Could you check a few things on this model? Use its own coordinates, in mm. A direction names the side the tool comes from. Give positions to 0.01 mm unless a question says otherwise; leave off trailing zeros. Order: outer loops, then holes, each group sorted by start corner. A loop starts at its lowest first (then second) coordinate and runs counter-clockwise, first axis right, second up.
from build123d import *

# Parameters (mm, degrees)
ESQUISSE1_W                                    = 408.5
ESQUISSE1_H                                    = 181
BOSS_EXTRU_1_DEPTH                             = 8
CHAMBRAGE_POUR_VIS_T_TE_RONDE_BOMB_2_COUNT     = 2
CHAMBRAGE_POUR_VIS_T_TE_RONDE_BOMB_2_PITCH     = 56
CHAMBRAGE_POUR_VIS_T_TE_RONDE_BOMB_3_COUNT     = 2
CHAMBRAGE_POUR_VIS_T_TE_RONDE_BOMB_3_PITCH     = 140
R_P_TITION_LIN_AIRE1_COUNT                     = 11
R_P_TITION_LIN_AIRE1_PITCH                     = 33
ESQUISSE4_W                                    = 22.5
ESQUISSE4_H                                    = 4.5
ENL_V_MAT_EXTRU_1_DEPTH                        = 181
ESQUISSE5_W                                    = 22.5
ESQUISSE5_H                                    = 18.725
BOSS_EXTRU_2_DEPTH                             = 3.5
ESQUISSE7_W                                    = 274.5
ESQUISSE7_H                                    = 22.375
BOSS_EXTRU_3_DEPTH                             = 5
FRAISAGE_POUR_VIS_T_TE_FRAIS_E_M31_D           = 3.4
FRAISAGE_POUR_VIS_T_TE_FRAIS_E_M31_CSINK_D     = 6.3
FRAISAGE_POUR_VIS_T_TE_FRAIS_E_M31_CSINK_ANGLE = 90


with BuildPart() as part:
    # Esquisse1 → Boss.-Extru.1 (new body)
    with BuildSketch(Plane.XY):
        Rectangle(ESQUISSE1_W, ESQUISSE1_H)
    extrude(amount=BOSS_EXTRU_1_DEPTH)

    # Esquisse3 → Chambrage pour vis à tête ronde bombée M31 (revolve, cut)
    with BuildSketch(Plane(origin=(-156.75, 63, 8), x_dir=(0, -1, 0), z_dir=(1, 0, 0))):
        Polygon((0, 0), (0, 8), (1.6, 8), (1.6, 2.4), (3.5, 2.4), (3.5, 0.025), (3.525, 0), align=None)
    chambrage_pour_vis_t_te_ronde_bomb_e_m = revolve(axis=Axis((-156.75, 63, 14.35), (0, 0, -1)), mode=Mode.SUBTRACT)

    # Chambrage pour vis _ t_te ronde bomb 2: Chambrage pour vis à tête ronde bombée M31 ×2
    with Locations(*[(0, -i * CHAMBRAGE_POUR_VIS_T_TE_RONDE_BOMB_2_PITCH, 0) for i in range(1, CHAMBRAGE_POUR_VIS_T_TE_RONDE_BOMB_2_COUNT)]):
        add(chambrage_pour_vis_t_te_ronde_bomb_e_m, mode=Mode.SUBTRACT)

    # Chambrage pour vis _ t_te ronde bomb 3: Chambrage pour vis à tête ronde bombée M31 ×2
    with Locations(*[(0, -i * CHAMBRAGE_POUR_VIS_T_TE_RONDE_BOMB_3_PITCH, 0) for i in range(1, CHAMBRAGE_POUR_VIS_T_TE_RONDE_BOMB_3_COUNT)]):
        add(chambrage_pour_vis_t_te_ronde_bomb_e_m, mode=Mode.SUBTRACT)

    # Répétition linéaire1: Chambrage pour vis à tête ronde bombée M31 ×11
    with Locations(*[(i * R_P_TITION_LIN_AIRE1_PITCH, 0, 0) for i in range(1, R_P_TITION_LIN_AIRE1_COUNT)]):
        add(chambrage_pour_vis_t_te_ronde_bomb_e_m, mode=Mode.SUBTRACT)

    # Répétition linéaire1 copy 1 sketch → Répétition linéaire1 copy 1 (revolve, cut)
    with BuildSketch(Plane(origin=(-123.75, 7, 8), x_dir=(0, -1, 0), z_dir=(1, 0, 0))):
        Polygon((0, 0), (0, 8), (1.6, 8), (1.6, 2.4), (3.5, 2.4), (3.5, 0.025), (3.525, 0), align=None)
    revolve(axis=Axis((-123.75, 7, 14.35), (0, 0, -1)), mode=Mode.SUBTRACT)

    # Répétition linéaire1 copy 2 sketch → Répétition linéaire1 copy 2 (revolve, cut)
    with BuildSketch(Plane(origin=(-90.75, 7, 8), x_dir=(0, -1, 0), z_dir=(1, 0, 0))):
        Polygon((0, 0), (0, 8), (1.6, 8), (1.6, 2.4), (3.5, 2.4), (3.5, 0.025), (3.525, 0), align=None)
    revolve(axis=Axis((-90.75, 7, 14.35), (0, 0, -1)), mode=Mode.SUBTRACT)

    # Répétition linéaire1 copy 3 sketch → Répétition linéaire1 copy 3 (revolve, cut)
    with BuildSketch(Plane(origin=(-57.75, 7, 8), x_dir=(0, -1, 0), z_dir=(1, 0, 0))):
        Polygon((0, 0), (0, 8), (1.6, 8), (1.6, 2.4), (3.5, 2.4), (3.5, 0.025), (3.525, 0), align=None)
    revolve(axis=Axis((-57.75, 7, 14.35), (0, 0, -1)), mode=Mode.SUBTRACT)

    # Répétition linéaire1 copy 4 sketch → Répétition linéaire1 copy 4 (revolve, cut)
    with BuildSketch(Plane(origin=(-24.75, 7, 8), x_dir=(0, -1, 0), z_dir=(1, 0, 0))):
        Polygon((0, 0), (0, 8), (1.6, 8), (1.6, 2.4), (3.5, 2.4), (3.5, 0.025), (3.525, 0), align=None)
    revolve(axis=Axis((-24.75, 7, 14.35), (0, 0, -1)), mode=Mode.SUBTRACT)

    # Répétition linéaire1 copy 5 sketch → Répétition linéaire1 copy 5 (revolve, cut)
    with BuildSketch(Plane(origin=(8.25, 7, 8), x_dir=(0, -1, 0), z_dir=(1, 0, 0))):
        Polygon((0, 0), (0, 8), (1.6, 8), (1.6, 2.4), (3.5, 2.4), (3.5, 0.025), (3.525, 0), align=None)
    revolve(axis=Axis((8.25, 7, 14.35), (0, 0, -1)), mode=Mode.SUBTRACT)

    # Répétition linéaire1 copy 6 sketch → Répétition linéaire1 copy 6 (revolve, cut)
    with BuildSketch(Plane(origin=(41.25, 7, 8), x_dir=(0, -1, 0), z_dir=(1, 0, 0))):
        Polygon((0, 0), (0, 8), (1.6, 8), (1.6, 2.4), (3.5, 2.4), (3.5, 0.025), (3.525, 0), align=None)
    revolve(axis=Axis((41.25, 7, 14.35), (0, 0, -1)), mode=Mode.SUBTRACT)

    # Répétition linéaire1 copy 7 sketch → Répétition linéaire1 copy 7 (revolve, cut)
    with BuildSketch(Plane(origin=(74.25, 7, 8), x_dir=(0, -1, 0), z_dir=(1, 0, 0))):
        Polygon((0, 0), (0, 8), (1.6, 8), (1.6, 2.4), (3.5, 2.4), (3.5, 0.025), (3.525, 0), align=None)
    revolve(axis=Axis((74.25, 7, 14.35), (0, 0, -1)), mode=Mode.SUBTRACT)

    # Répétition linéaire1 copy 8 sketch → Répétition linéaire1 copy 8 (revolve, cut)
    with BuildSketch(Plane(origin=(107.25, 7, 8), x_dir=(0, -1, 0), z_dir=(1, 0, 0))):
        Polygon((0, 0), (0, 8), (1.6, 8), (1.6, 2.4), (3.5, 2.4), (3.5, 0.025), (3.525, 0), align=None)
    revolve(axis=Axis((107.25, 7, 14.35), (0, 0, -1)), mode=Mode.SUBTRACT)

    # Répétition linéaire1 copy 9 sketch → Répétition linéaire1 copy 9 (revolve, cut)
    with BuildSketch(Plane(origin=(140.25, 7, 8), x_dir=(0, -1, 0), z_dir=(1, 0, 0))):
        Polygon((0, 0), (0, 8), (1.6, 8), (1.6, 2.4), (3.5, 2.4), (3.5, 0.025), (3.525, 0), align=None)
    revolve(axis=Axis((140.25, 7, 14.35), (0, 0, -1)), mode=Mode.SUBTRACT)

    # Répétition linéaire1 copy 10 sketch → Répétition linéaire1 copy 10 (revolve, cut)
    with BuildSketch(Plane(origin=(173.25, 7, 8), x_dir=(0, -1, 0), z_dir=(1, 0, 0))):
        Polygon((0, 0), (0, 8), (1.6, 8), (1.6, 2.4), (3.5, 2.4), (3.5, 0.025), (3.525, 0), align=None)
    revolve(axis=Axis((173.25, 7, 14.35), (0, 0, -1)), mode=Mode.SUBTRACT)

    # Répétition linéaire1 copy 11 sketch → Répétition linéaire1 copy 11 (revolve, cut)
    with BuildSketch(Plane(origin=(-123.75, -77, 8), x_dir=(0, -1, 0), z_dir=(1, 0, 0))):
        Polygon((0, 0), (0, 8), (1.6, 8), (1.6, 2.4), (3.5, 2.4), (3.5, 0.025), (3.525, 0), align=None)
    revolve(axis=Axis((-123.75, -77, 14.35), (0, 0, -1)), mode=Mode.SUBTRACT)

    # Répétition linéaire1 copy 12 sketch → Répétition linéaire1 copy 12 (revolve, cut)
    with BuildSketch(Plane(origin=(-90.75, -77, 8), x_dir=(0, -1, 0), z_dir=(1, 0, 0))):
        Polygon((0, 0), (0, 8), (1.6, 8), (1.6, 2.4), (3.5, 2.4), (3.5, 0.025), (3.525, 0), align=None)
    revolve(axis=Axis((-90.75, -77, 14.35), (0, 0, -1)), mode=Mode.SUBTRACT)

    # Répétition linéaire1 copy 13 sketch → Répétition linéaire1 copy 13 (revolve, cut)
    with BuildSketch(Plane(origin=(-57.75, -77, 8), x_dir=(0, -1, 0), z_dir=(1, 0, 0))):
        Polygon((0, 0), (0, 8), (1.6, 8), (1.6, 2.4), (3.5, 2.4), (3.5, 0.025), (3.525, 0), align=None)
    revolve(axis=Axis((-57.75, -77, 14.35), (0, 0, -1)), mode=Mode.SUBTRACT)

    # Répétition linéaire1 copy 14 sketch → Répétition linéaire1 copy 14 (revolve, cut)
    with BuildSketch(Plane(origin=(-24.75, -77, 8), x_dir=(0, -1, 0), z_dir=(1, 0, 0))):
        Polygon((0, 0), (0, 8), (1.6, 8), (1.6, 2.4), (3.5, 2.4), (3.5, 0.025), (3.525, 0), align=None)
    revolve(axis=Axis((-24.75, -77, 14.35), (0, 0, -1)), mode=Mode.SUBTRACT)

    # Répétition linéaire1 copy 15 sketch → Répétition linéaire1 copy 15 (revolve, cut)
    with BuildSketch(Plane(origin=(8.25, -77, 8), x_dir=(0, -1, 0), z_dir=(1, 0, 0))):
        Polygon((0, 0), (0, 8), (1.6, 8), (1.6, 2.4), (3.5, 2.4), (3.5, 0.025), (3.525, 0), align=None)
    revolve(axis=Axis((8.25, -77, 14.35), (0, 0, -1)), mode=Mode.SUBTRACT)

    # Répétition linéaire1 copy 16 sketch → Répétition linéaire1 copy 16 (revolve, cut)
    with BuildSketch(Plane(origin=(41.25, -77, 8), x_dir=(0, -1, 0), z_dir=(1, 0, 0))):
        Polygon((0, 0), (0, 8), (1.6, 8), (1.6, 2.4), (3.5, 2.4), (3.5, 0.025), (3.525, 0), align=None)
    revolve(axis=Axis((41.25, -77, 14.35), (0, 0, -1)), mode=Mode.SUBTRACT)

    # Répétition linéaire1 copy 17 sketch → Répétition linéaire1 copy 17 (revolve, cut)
    with BuildSketch(Plane(origin=(74.25, -77, 8), x_dir=(0, -1, 0), z_dir=(1, 0, 0))):
        Polygon((0, 0), (0, 8), (1.6, 8), (1.6, 2.4), (3.5, 2.4), (3.5, 0.025), (3.525, 0), align=None)
    revolve(axis=Axis((74.25, -77, 14.35), (0, 0, -1)), mode=Mode.SUBTRACT)

    # Répétition linéaire1 copy 18 sketch → Répétition linéaire1 copy 18 (revolve, cut)
    with BuildSketch(Plane(origin=(107.25, -77, 8), x_dir=(0, -1, 0), z_dir=(1, 0, 0))):
        Polygon((0, 0), (0, 8), (1.6, 8), (1.6, 2.4), (3.5, 2.4), (3.5, 0.025), (3.525, 0), align=None)
    revolve(axis=Axis((107.25, -77, 14.35), (0, 0, -1)), mode=Mode.SUBTRACT)

    # Répétition linéaire1 copy 19 sketch → Répétition linéaire1 copy 19 (revolve, cut)
    with BuildSketch(Plane(origin=(140.25, -77, 8), x_dir=(0, -1, 0), z_dir=(1, 0, 0))):
        Polygon((0, 0), (0, 8), (1.6, 8), (1.6, 2.4), (3.5, 2.4), (3.5, 0.025), (3.525, 0), align=None)
    revolve(axis=Axis((140.25, -77, 14.35), (0, 0, -1)), mode=Mode.SUBTRACT)

    # Répétition linéaire1 copy 20 sketch → Répétition linéaire1 copy 20 (revolve, cut)
    with BuildSketch(Plane(origin=(173.25, -77, 8), x_dir=(0, -1, 0), z_dir=(1, 0, 0))):
        Polygon((0, 0), (0, 8), (1.6, 8), (1.6, 2.4), (3.5, 2.4), (3.5, 0.025), (3.525, 0), align=None)
    revolve(axis=Axis((173.25, -77, 14.35), (0, 0, -1)), mode=Mode.SUBTRACT)

    # Esquisse4 → Enlèv. mat.-Extru.1 (cut)
    with BuildSketch(Plane(origin=(0, 90.5, 0), x_dir=(1, 0, 0), z_dir=(0, 1, 0))):
        with Locations((-193, -2.25)):
            Rectangle(ESQUISSE4_W, ESQUISSE4_H)
        with Locations((193, -2.25)):
            Rectangle(ESQUISSE4_W, ESQUISSE4_H)
    extrude(amount=-ENL_V_MAT_EXTRU_1_DEPTH, mode=Mode.SUBTRACT)

    # Esquisse5 → Boss.-Extru.2 (add)
    with BuildSketch(Plane.XY.offset(8)):
        with Locations((-193, 99.8625)):
            Rectangle(ESQUISSE5_W, ESQUISSE5_H)
    boss_extru_2 = extrude(amount=-BOSS_EXTRU_2_DEPTH)

    # Symétrie1: Boss.-Extru.2 across plane
    add(boss_extru_2.mirror(Plane(origin=(0, 0, 0), x_dir=(0, 0, 1), z_dir=(1, 0, 0))))

    # Esquisse7 → Boss.-Extru.3 (add)
    with BuildSketch(Plane.XY.offset(8)):
        with Locations((0, 101.6875)):
            Rectangle(ESQUISSE7_W, ESQUISSE7_H)
    extrude(amount=-BOSS_EXTRU_3_DEPTH)

    # Fraisage pour vis à tête fraisée M31 (through all)
    with Locations(Plane.XY.offset(8)):
        with Locations((-131.25, 98), (131.25, 98)):
            CounterSinkHole(FRAISAGE_POUR_VIS_T_TE_FRAIS_E_M31_D / 2, FRAISAGE_POUR_VIS_T_TE_FRAIS_E_M31_CSINK_D / 2, counter_sink_angle=FRAISAGE_POUR_VIS_T_TE_FRAIS_E_M31_CSINK_ANGLE)


solid = part.part
Item 1: For pin 1 (6.5 mm diameter, centred on x = 41.25, y = 7, fed in from -Z); pin 2 (2 mm diameter, centred on y = 33.5, z = 3, fed in from -X); pin 3 (3.5 mm diameter, centred on x = 173, y = 7, fed in from +Z), each with a flat end and sliding along its axis, tell me the tip position at first contact or that it passes through.
Findings:
pin 1: stops at z = 0
pin 2: stops at x = -181.75
pin 3: stops at z = 5.6
Item 2: Please list where these lines run through material, in increasing order: line 1 along Y through (x, z) = (-57.5, 6) (3 decimals); line 2 along Y through (x, z) = (-90.75, 3.9) (3 decimals); line 3 along Y through (x, z) = (131.25, 5.3) (3 decimals).
Findings:
line 1: y = -90.5 to -80.491, -73.509 to 3.509, 10.491 to 59.509, 66.491 to 112.875
line 2: y = -90.5 to -78.6, -75.4 to 5.4, 8.6 to 61.4, 64.6 to 112.875
line 3: y = -90.5 to 96.3, 99.7 to 112.875
Item 3: Imagine slicing it at A-A on y = -54.5. List the corners of the cut face in (x, z) for me, then the cut area to 3 significant figures.
Findings:
outline: (-204.25, 4.5) - (-181.75, 4.5) - (-181.75, 0) - (181.75, 0) - (181.75, 4.5) - (204.25, 4.5) - (204.25, 8) - (-204.25, 8) - close
area: 3,070 mm2
Item 4: Imagine slicing it at B-B on x = 82. List the corners of the cut face in (y, z) for me (3 decimals).
Findings:
outline: (-90.5, 0) - (90.5, 0) - (90.5, 3) - (112.875, 3) - (112.875, 8) - (-90.5, 8) - close
Item 5: For faces 4 (the flat face through (-56, 8, 5.6)), 5 (the flat face through (-2, 102, 3)), which set-ups out of +Z, -Z, +X, -X, +Y, -Y let a thin tool reach every point of the face, with its end or its side?
Findings:
face 4: +Z
face 5: -Z, +X, -X, +Y
Item 6: We'd pull the mould along Y, two halves only. Please class faces 1 (the flat face through (-123, -75, 5.6)), 2 (the flat face through (-3, 90.5, 2)), 3 (the flat face through (-3, 1, 0)): +Y half, -Y half, draft (parallel to the pull), parting line (faces both ways), or undercut.
Findings:
face 1: undercut
face 2: +Y half
face 3: draft
